CAD build for the part. Positions are in the model's coordinates, mm. A direction names the side the tool comes from. Give positions to 0.01 mm unless a question says otherwise; leave off trailing zeros. Loops run counter-clockwise (first coordinate to the right, second up) from the corner with the lowest first, then second, coordinate; pieces in that order, holes last. Notation, with made-up numbers: (13, -36.5) - (19, -36.5) arc R26 cw to (19, -13.5) - close; hole circle Ø4 at (-36, -25). An arc over 180 degrees is marked (long way). Return JSON: item names as keys, results as strings.
from build123d import *

# Parameters (mm, degrees)
BLANKSKE_W          = 53
BLANKSKE_H          = 8.2
BLANK_DEPTH         = 5
TOOTHCUTSIM_DEPTH   = 54.863159952
TEETHCUTS_COUNT     = 18
TEETHCUTS_PITCH     = 3.14159265
SKETCH2_W           = 6.72762067
SKETCH2_H           = 5.95
BOSS_EXTRUDE1_DEPTH = 20
SKETCH3_W           = 12
SKETCH3_H           = 5.95
BOSS_EXTRUDE2_DEPTH = 16
SKETCH4_W           = 6.72762067
SKETCH4_H           = 5.95
CUT_EXTRUDE1_DEPTH  = 4
SKETCH7_W           = 12.002
SKETCH7_H           = 8.2
CUT_EXTRUDE3_DEPTH  = 9.55
SKETCH9_W           = 1.263
SKETCH9_H           = 21
CUT_EXTRUDE4_DEPTH  = 9.55
SKETCH10_W          = 4.57574993
SKETCH10_H          = 2.726704985
CUT_EXTRUDE6_DEPTH  = 9.55
BLANKSKE_2_W        = 53
BLANKSKE_2_H        = 8.2
CUT_EXTRUDE7_DEPTH  = 0.1
SKETCH11_W          = 34.27037933
SKETCH11_H          = 11.830057098
CUT_EXTRUDE8_DEPTH  = 0.1


with BuildPart() as part:
    # BlankSke → Blank (new body)
    with BuildSketch(Plane.XY):
        with Locations((26.5, 4.1)):
            Rectangle(BLANKSKE_W, BLANKSKE_H)
    extrude(amount=-BLANK_DEPTH)

    # TooCutSkeSim → ToothCutSim (cut, through all)
    with BuildSketch(Plane.XY):
        Polygon((0.44443537, 5.95), (-0.44443537, 5.95), (-1.272613241, 8.2254), (1.272613241, 8.2254), align=None)
    toothcutsim = extrude(amount=-TOOTHCUTSIM_DEPTH, mode=Mode.SUBTRACT)

    # TeethCuts: ToothCutSim ×18
    with Locations(*[(i * TEETHCUTS_PITCH, 0, 0) for i in range(1, TEETHCUTS_COUNT)]):
        add(toothcutsim, mode=Mode.SUBTRACT)

    # Sketch2 → Boss-Extrude1 (add)
    with BuildSketch(Plane(origin=(0, 0, -5), x_dir=(-1, 0, 0), z_dir=(0, 0, -1))):
        with Locations((-3.363810335, 2.975)):
            Rectangle(SKETCH2_W, SKETCH2_H)
    extrude(amount=BOSS_EXTRUDE1_DEPTH)

    # Sketch3 → Boss-Extrude2 (add)
    with BuildSketch(Plane(origin=(6.72762067, 0, 0), x_dir=(0, 0, -1), z_dir=(1, 0, 0))):
        with Locations((15, 2.975)):
            Rectangle(SKETCH3_W, SKETCH3_H)
    extrude(amount=BOSS_EXTRUDE2_DEPTH)

    # Sketch4 → Cut-Extrude1 (cut)
    with BuildSketch(Plane(origin=(0, 0, -25), x_dir=(-1, 0, 0), z_dir=(0, 0, -1))):
        with Locations((-3.363810335, 2.975)):
            Rectangle(SKETCH4_W, SKETCH4_H)
    extrude(amount=-CUT_EXTRUDE1_DEPTH, mode=Mode.SUBTRACT)

    # Sketch7 → Cut-Extrude3 (cut)
    with BuildSketch(Plane(origin=(0, 0, -5), x_dir=(-1, 0, 0), z_dir=(0, 0, -1))):
        with Locations((-46.999, 4.1)):
            Rectangle(SKETCH7_W, SKETCH7_H)
    extrude(amount=-CUT_EXTRUDE3_DEPTH, mode=Mode.SUBTRACT)

    # Sketch9 → Cut-Extrude4 (cut)
    with BuildSketch(Plane.XZ):
        with Locations((0.6315, -10.5)):
            Rectangle(SKETCH9_W, SKETCH9_H)
    extrude(amount=-CUT_EXTRUDE4_DEPTH, mode=Mode.SUBTRACT)

    # Sketch10 → Cut-Extrude6 (cut)
    with BuildSketch(Plane.XY):
        with Locations((3.550874965, 7.313352492)):
            Rectangle(SKETCH10_W, SKETCH10_H)
    extrude(amount=-CUT_EXTRUDE6_DEPTH, mode=Mode.SUBTRACT)

    # BlankSke<2> → Cut-Extrude7 (cut)
    with BuildSketch(Plane.XY):
        with Locations((26.5, 4.1)):
            Rectangle(BLANKSKE_2_W, BLANKSKE_2_H)
    extrude(amount=-CUT_EXTRUDE7_DEPTH, mode=Mode.SUBTRACT)

    # Sketch11 → Cut-Extrude8 (cut)
    with BuildSketch(Plane(origin=(0, 0, -5), x_dir=(-1, 0, 0), z_dir=(0, 0, -1))):
        with Locations((-23.862810335, 5.915028549)):
            Rectangle(SKETCH11_W, SKETCH11_H)
    extrude(amount=-CUT_EXTRUDE8_DEPTH, mode=Mode.SUBTRACT)


solid = part.part
1. Which spindle directions (+Z, -Z, +X, -X, +Y, -Y) get a long thin tool onto all of the face, cutting with end or side? Do faces 1 (the face through (22.728, 3, -15)), 2 (the face through (25.99, 7.09, -2.47)), 3 (the face through (40.998, 3, -3)). Say none if no direction does.
Values follow:
{"face 1": "-Z, +X, +Y, -Y", "face 2": "+Z, -Z, +Y", "face 3": "+Z, -Z, +X, +Y, -Y"}
2. Cut at A-A, the plane y = 4.75. Write the cut outline in (x, z).
Values follow:
{"outline": "(1.26, -21) - (22.73, -21) - (22.73, -9) - (6.73, -9) - (6.73, -4.9) - (41, -4.9) - (41, -0.1) - (1.26, -0.1) - close"}
3. Cut at B-B, the plane z = -10. Write the cut outline in (x, y), plus the area to 3 significant figures.
Values follow:
{"outline": "(1.26, 0) - (22.73, 0) - (22.73, 5.95) - (1.26, 5.95) - close", "area": "128 mm²"}
4. Pull direction X, two halves, no side cores. Call faces 4 (the face through (17, 0, -10)), 5 (the face through (39.993, 7.059, -2.466)), 6 (the face through (37.7, 5.95, -2.5)): +X half, -X half, draft (parallel to the pull), parting line (faces both ways), or undercut.
Values follow:
{"face 4": "draft", "face 5": "+X half", "face 6": "undercut"}
5. Drop flat-ended pins along their axis: P1, Ø6, axis at x = 16.5, z = -3, coming from the +Y side; P2, Ø1, axis at y = 1, z = -7.5, coming from the +X side; P3, Ø2, axis at x = 15, z = -15.5, coming from the +Y side; P4, Ø10, axis at x = 33, z = -10, coming from the +Y side. Give the stop position or say it passes through.
Values follow:
{"P1": "stops at y = 8.2", "P2": "stops at x = 6.73", "P3": "stops at y = 5.95", "P4": "passes through"}
6. Drill centre lines: probe 1 along Z at (x, y) = (9, 4.25); probe 2 along Y at (x, z) = (5.5, -4.25); probe 3 along X at (y, z) = (5.25, -14.25). Where is each one in solid material? Low to high.
Values follow:
{"probe 1": "z = -21 to -9, -4.9 to -0.1", "probe 2": "y = 0 to 5.95", "probe 3": "x = 1.26 to 22.73"}
